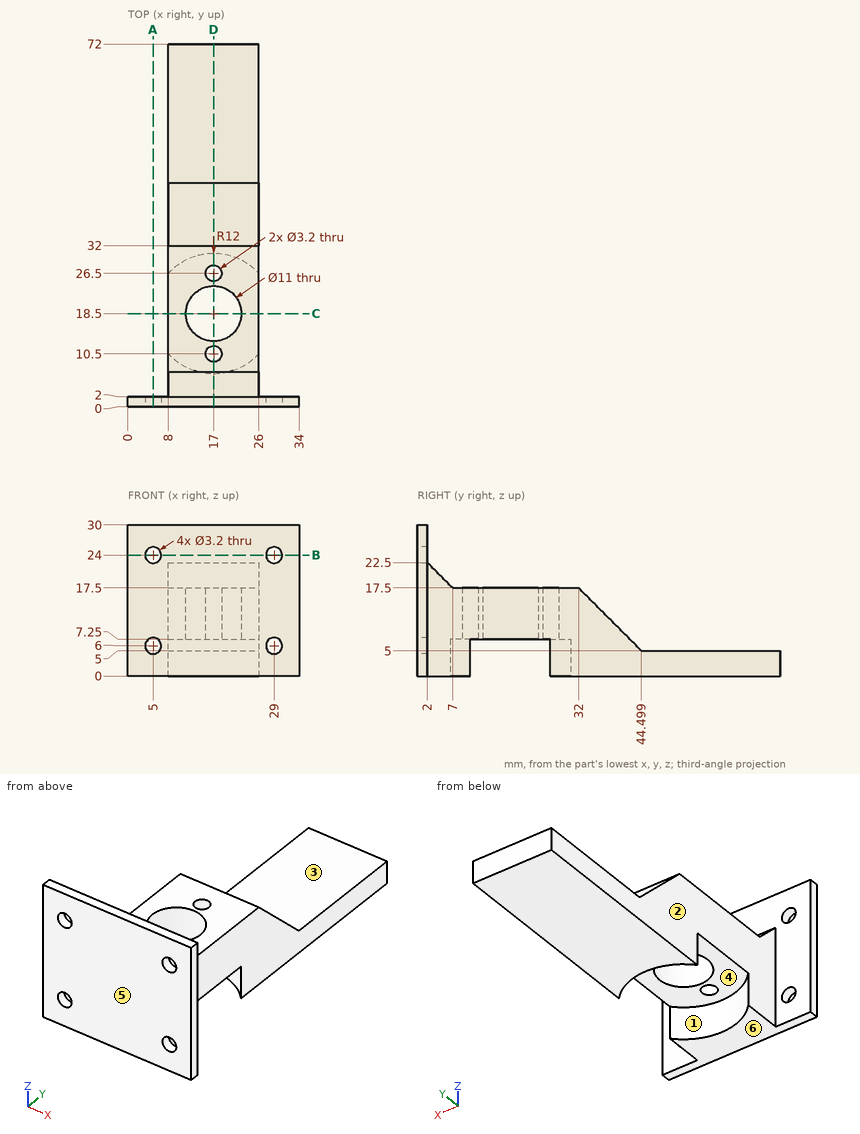
Drawing for the job (mm, zero at the part's lowest x, y, z). A direction names the side the tool comes from. Give positions to 0.01 mm unless a question says otherwise; leave off trailing zeros. Loops run counter-clockwise (first coordinate to the right, second up) from the corner with the lowest first, then second, coordinate; pieces in that order, holes last. Notation, with made-up numbers: (47, -11.75) - (96, -11.75) arc R13 ccw to (96, -3.75) - close; hole circle Ø2 at (3.25, -26.75). An arc over 180 degrees is marked (long way). Write item = value, one per line. Start each with the question number.
1) Band-saw the part on B-B on z = 24. Give the cut face in (x, y).
2) Pull direction Y, two halves, no side cores. Call the marked faces 4, 5 and 6: +Y half, -Y half, draft (parallel to the pull), parting line (faces both ways), or undercut.
3) Drop flat-ended pins along their axis: pin 1 Ø5 at (x, y) = (17, 10.5) entering from +Z; pin 2 Ø1.9 at (x, z) = (29, 24) entering from +Y; pin 3 Ø4 at (y, z) = (34, 12.5) entering from -X; pin 4 Ø5.5 at (x, y) = (15.5, 57) entering from +Z. Give the stop position or say it passes through.
4) Band-saw the part on C-C on y = 18.5. Give the cut face in (x, z).
5) Tool access for the marked faces 1, 2 and 3: list every direction of +Z, -Z, +X, -X, +Y, -Y with a clear straight run to the whole face (end or side of a thin tool).
6) Band-saw the part on A-A on x = 5. Give the cut face in (y, z).
7) Band-saw the part on D-D on x = 17. Count the separate pieces of the cut face and the enclosed holes in it.
8) Probe probe 1 along Z at (x, y) = (5, 0.85); probe 2 along X at (y, z) = (1.45, 24); probe 3 along Z at (x, y) = (18, 50.5). List the from-to ranges inside material, lowest first. Write a range as from..to.
Final values:
q1.outline = (0, 0) - (3.4, 0) - (3.4, 2) - (0, 2) - close; (6.6, 0) - (27.4, 0) - (27.4, 2) - (6.6, 2) - close; (30.6, 0) - (34, 0) - (34, 2) - (30.6, 2) - close
q2.face_4 = undercut
q2.face_5 = -Y half
q2.face_6 = draft
q3.pin_1 = 17.5
q3.pin_2 = through
q3.pin_3 = 8
q3.pin_4 = 5
q4.outline = (8, 7.25) - (11.5, 7.25) - (11.5, 17.5) - (8, 17.5) - close; (22.5, 7.25) - (26, 7.25) - (26, 17.5) - (22.5, 17.5) - close
q5.face_1 = -Z
q5.face_2 = +Z, -Z, -X, +Y
q5.face_3 = +Z, +X, -X, +Y
q6.outline = (0, 0) - (2, 0) - (2, 4.4) - (0, 4.4) - close; (0, 7.6) - (2, 7.6) - (2, 22.4) - (0, 22.4) - close; (0, 25.6) - (2, 25.6) - (2, 30) - (0, 30) - close
q7.separate_pieces = 4
q7.enclosed_holes = 0
q8.probe_1 = 0..4.4, 7.6..22.4, 25.6..30
q8.probe_2 = 0..3.4, 6.6..27.4, 30.6..34
q8.probe_3 = 0..5
